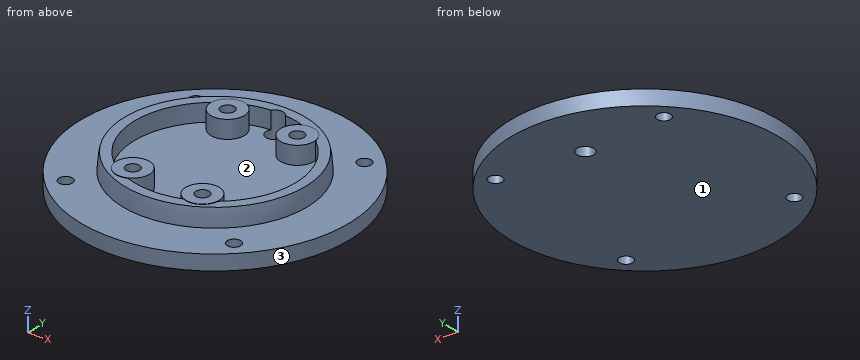
```python
from build123d import *

# Parameters (mm, degrees)
CYLINDER170_R             = 2
CYLINDER170_DEPTH         = 10
CYLINDER171_R             = 2
CYLINDER171_DEPTH         = 10
CYLINDER172_R             = 2
CYLINDER172_DEPTH         = 10
CYLINDER169_R             = 2
CYLINDER169_DEPTH         = 10
FUSION111_PLACEMENT_ANGLE = 45
CYLINDER165_R             = 2.5
CYLINDER165_DEPTH         = 60
CYLINDER161_R             = 2
CYLINDER161_DEPTH         = 10
CYLINDER162_R             = 2
CYLINDER162_DEPTH         = 10
CYLINDER163_R             = 2
CYLINDER163_DEPTH         = 10
CYLINDER164_R             = 2
CYLINDER164_DEPTH         = 10
CYLINDER156_R             = 5.5
CYLINDER156_DEPTH         = 1
CYLINDER157_R             = 5
CYLINDER157_DEPTH         = 5.82
CYLINDER158_R             = 5
CYLINDER158_DEPTH         = 5.82
CYLINDER159_R             = 5
CYLINDER159_DEPTH         = 5.82
CYLINDER160_R             = 5
CYLINDER160_DEPTH         = 5.82
CYLINDER154_R             = 40
CYLINDER154_DEPTH         = 4.5
CYLINDER155_R             = 24
CYLINDER155_DEPTH         = 7


with BuildPart() as obj1:
    # Cylinder170 → Cylinder170 (new body)
    with BuildSketch(Plane(origin=(35, 0, 65), x_dir=(1, 0, 0), z_dir=(0, 0, 1))):
        Circle(CYLINDER170_R)
    extrude(amount=CYLINDER170_DEPTH)


with BuildPart() as obj2:
    # Cylinder171 → Cylinder171 (new body)
    with BuildSketch(Plane(origin=(0, 35, 65), x_dir=(1, 0, 0), z_dir=(0, 0, 1))):
        Circle(CYLINDER171_R)
    extrude(amount=CYLINDER171_DEPTH)


with BuildPart() as obj3:
    # Cylinder172 → Cylinder172 (new body)
    with BuildSketch(Plane(origin=(0, -35, 65), x_dir=(1, 0, 0), z_dir=(0, 0, 1))):
        Circle(CYLINDER172_R)
    extrude(amount=CYLINDER172_DEPTH)


with BuildPart() as fusion111:
    # Cylinder169 → Cylinder169 (new body)
    with BuildSketch(Plane(origin=(-35, 0, 65), x_dir=(1, 0, 0), z_dir=(0, 0, 1))):
        Circle(CYLINDER169_R)
    extrude(amount=CYLINDER169_DEPTH)

    # Fusion111: union obj1, obj2, obj3
    add(obj1.part)
    add(obj2.part)
    add(obj3.part)


with BuildPart() as fusion111_1:
    # Fusion111 placement: moved
    add(fusion111.part.moved(Location((0, -374, -75))).rotate(Axis((0, -374, -75), (0, 0, -1)), FUSION111_PLACEMENT_ANGLE))


with BuildPart() as wirecut004:
    # Cylinder165 → Cylinder165 (new body)
    with BuildSketch(Plane(origin=(134, 32.6, 20), x_dir=(1, 0, 0), z_dir=(0, 0, 1))):
        Circle(CYLINDER165_R)
    extrude(amount=CYLINDER165_DEPTH)


with BuildPart() as cylinder161:
    # Cylinder161 → Cylinder161 (new body)
    with BuildSketch(Plane(origin=(0, -21, 0), x_dir=(1, 0, 0), z_dir=(0, 0, 1))):
        Circle(CYLINDER161_R)
    extrude(amount=CYLINDER161_DEPTH)


with BuildPart() as m3heatsetcuts025:
    # Cylinder162 → Cylinder162 (new body)
    with BuildSketch(Plane(origin=(20.5, -21, 0), x_dir=(1, 0, 0), z_dir=(0, 0, 1))):
        Circle(CYLINDER162_R)
    extrude(amount=CYLINDER162_DEPTH)

    # Fusion103: union Cylinder161
    add(cylinder161.part)


with BuildPart() as m3heatsetcuts025_1:
    # Fusion103 placement: moved
    add(m3heatsetcuts025.part.moved(Location((-5, 39, 70))))


with BuildPart() as cylinder163:
    # Cylinder163 → Cylinder163 (new body)
    with BuildSketch(Plane(origin=(0, -21, 0), x_dir=(1, 0, 0), z_dir=(0, 0, 1))):
        Circle(CYLINDER163_R)
    extrude(amount=CYLINDER163_DEPTH)


with BuildPart() as lightmodulecut005:
    # Cylinder164 → Cylinder164 (new body)
    with BuildSketch(Plane(origin=(20.5, -21, 0), x_dir=(1, 0, 0), z_dir=(0, 0, 1))):
        Circle(CYLINDER164_R)
    extrude(amount=CYLINDER164_DEPTH)

    # Fusion104: union Cylinder163
    add(cylinder163.part)


with BuildPart() as lightmodulecut005_1:
    # Fusion104 placement: moved
    add(lightmodulecut005.part.moved(Location((-5, 3, 70))))

    # Fusion102: union m3HeatSetCuts025
    add(m3heatsetcuts025_1.part)


with BuildPart() as lightmodulecut005_2:
    # Fusion102 placement: moved
    add(lightmodulecut005_1.part.moved(Location((128.75, 10, -1))))

    # Fusion105: union WireCut004
    add(wirecut004.part)


with BuildPart() as cylinder156:
    # Cylinder156 → Cylinder156 (new body)
    with BuildSketch(Plane(origin=(134, 32.6, 65), x_dir=(1, 0, 0), z_dir=(0, 0, 1))):
        Circle(CYLINDER156_R)
    extrude(amount=CYLINDER156_DEPTH)


with BuildPart() as cylinder157:
    # Cylinder157 → Cylinder157 (new body)
    with BuildSketch(Plane(origin=(0, -21, 0), x_dir=(1, 0, 0), z_dir=(0, 0, 1))):
        Circle(CYLINDER157_R)
    extrude(amount=CYLINDER157_DEPTH)


with BuildPart() as m3heatsetcuts021:
    # Cylinder158 → Cylinder158 (new body)
    with BuildSketch(Plane(origin=(20.5, -21, 0), x_dir=(1, 0, 0), z_dir=(0, 0, 1))):
        Circle(CYLINDER158_R)
    extrude(amount=CYLINDER158_DEPTH)

    # Fusion097: union Cylinder157
    add(cylinder157.part)


with BuildPart() as m3heatsetcuts021_1:
    # Fusion097 placement: moved
    add(m3heatsetcuts021.part.moved(Location((-5, 39, 70))))


with BuildPart() as cylinder159:
    # Cylinder159 → Cylinder159 (new body)
    with BuildSketch(Plane(origin=(0, -21, 0), x_dir=(1, 0, 0), z_dir=(0, 0, 1))):
        Circle(CYLINDER159_R)
    extrude(amount=CYLINDER159_DEPTH)


with BuildPart() as m3heatsetcuts023:
    # Cylinder160 → Cylinder160 (new body)
    with BuildSketch(Plane(origin=(20.5, -21, 0), x_dir=(1, 0, 0), z_dir=(0, 0, 1))):
        Circle(CYLINDER160_R)
    extrude(amount=CYLINDER160_DEPTH)

    # Fusion098: union Cylinder159
    add(cylinder159.part)


with BuildPart() as m3heatsetcuts023_1:
    # Fusion098 placement: moved
    add(m3heatsetcuts023.part.moved(Location((-5, 3, 70))))

    # Fusion099: union m3HeatSetCuts021
    add(m3heatsetcuts021_1.part)


with BuildPart() as m3heatsetcuts023_2:
    # Fusion099 placement: moved
    add(m3heatsetcuts023_1.part.moved(Location((128.75, 10, -1))))


with BuildPart() as base014:
    # Cylinder154 → Cylinder154 (new body)
    with BuildSketch(Plane(origin=(136, 0, 65), x_dir=(1, 0, 0), z_dir=(0, 0, 1))):
        Circle(CYLINDER154_R)
    extrude(amount=CYLINDER154_DEPTH)


with BuildPart() as basecut003:
    # Cylinder155 → Cylinder155 (new body)
    with BuildSketch(Plane(origin=(5, 0, 74), x_dir=(1, 0, 0), z_dir=(0, 0, 1))):
        Circle(CYLINDER155_R)
    extrude(amount=CYLINDER155_DEPTH)


with BuildPart() as cut058:
    # Sphere005 → Sphere005 (revolve)
    with BuildSketch(Plane(origin=(5, 0, 74), x_dir=(1, 0, 0), z_dir=(0, -1, 0))):
        with BuildLine():
            ThreePointArc((27.5, 0), (27.349352, 2.874533), (26.899059, 5.717571))
            Line((26.899059, 5.717571), (0, 5.717571))
            Line((0, 5.717571), (0, 0))
            Line((0, 0), (27.5, 0))
        make_face()
    revolve(axis=Axis((5, 0, 74), (0, 0, 1)))

    # Cut053: cut baseCut003
    add(basecut003.part, mode=Mode.SUBTRACT)


with BuildPart() as cut058_1:
    # Cut053 placement: moved
    add(cut058.part.moved(Location((131, 0, -5))))

    # Fusion100: union base014
    add(base014.part)


with BuildPart() as cut058_2:
    # Fusion100 placement: moved
    add(cut058_1.part.moved(Location((-2, 10, 0))))

    # Fusion101: union Cylinder156, m3HeatSetCuts023
    add(cylinder156.part)
    add(m3heatsetcuts023_2.part)

    # Cut054: cut lightModuleCut005
    add(lightmodulecut005_2.part, mode=Mode.SUBTRACT)


with BuildPart() as cut058_3:
    # Cut054 placement: moved
    add(cut058_2.part.moved(Location((-134, -384, -74))))

    # Cut058: cut Fusion111
    add(fusion111_1.part, mode=Mode.SUBTRACT)


solid = cut058_3.part
```
The listing builds one solid part. Answer for the finished solid, in the listing's coordinates (mm). Face numbers are marked on the shaded views. Give positions to 0.01 mm unless a question says otherwise; leave off trailing zeros. Loops run counter-clockwise (first coordinate to the right, second up) from the corner with the lowest first, then second, coordinate; pieces in that order, holes last. Notation, with made-up numbers: (-18, 11.5) - (32, 11.5) arc R26 cw to (32, 47.5) - close; hole circle Ø11 at (42.25, 16.25). An arc over 180 degrees is marked (long way). Answer as CSV lines item,"result". Start each with the question number.
Item 1: Find the intervals of material crossed by line 1 (X direction, y = -356, z = -3.65); line 2 (X direction, y = -398.5, z = -5); line 3 (Y direction, x = -10, z = 0), in increasing order. Write a range as from..to.
Item 2: A cutting plane is placed at C-C on x = -33. Determine the outline of the cut face in (y, z), then the cut area to 3 significant figures.
Item 3: Each of these flat-tipped pins is pushed along its axis until it touches: pin 1 (1.5 mm diameter, centred on y = -357.5, z = -7.5, fed in from +X); pin 2 (14.5 mm diameter, centred on x = -7.5, y = -368.5, fed in from +Z); pin 3 (1 mm diameter, centred on y = -363.5, z = -6.5, fed in from -X). Where does it stop, or does it pass through?
Item 4: A cutting plane is placed at B-B on y = -344.5. Determine the outline of the cut face in (x, z), then the cut area to 3 significant figures.
Item 5: A cutting plane is placed at A-A on z = -1. Count the separate pieces of the cut face and the enclosed holes in it, then the cut area to 3 significant figures.
Item 6: The mould has two halves that part along X. Classify the marked faces 1, 2 and 3: +X half, -X half, draft (parallel to the pull), parting line (faces both ways), or undercut.
Found:
1,line 1,"x = -20.75..-15.87, -15.25..-12.25, -8.25..-5.25, 5.25..8.25, 12.25..15.25, 15.87..20.75"
1,line 2,"x = -31.62..-26.73, -22.76..22.76, 26.73..31.62"
1,line 3,"y = -399.12..-393.98, -390.02..-387.01, -360.99..-357.98, -354.02..-348.88"
2,outline,"(-396.61, -9) - (-351.39, -9) - (-351.39, -4.5) - (-396.61, -4.5) - close"
2,area,"203 mm^2"
3,pin 1,"stops at x = 36.77"
3,pin 2,"stops at z = -4.5"
3,pin 3,"stops at x = -38.73"
4,outline,"(-27.01, -9) - (27.01, -9) - (27.01, -4.5) - (-27.01, -4.5) - close"
4,area,"243 mm^2"
5,separate pieces,"1"
5,enclosed holes,"5"
5,area,"737 mm^2"
6,face 1,"draft"
6,face 2,"undercut"
6,face 3,"parting line"
